For this review, use the dimensioned drawing (mm, ordinates from the lowest corner) and the shaded views. A direction names the side the tool comes from. Coordinates: 2 decimals unless noted, no trailing zeros. Loops run counter-clockwise (first coordinate to the right, second up) from the corner with the lowest first, then second, coordinate; pieces in that order, holes last. Notation, with made-up numbers: M 18,87.25 L 36,87.25 A21 cw 36,92.25 Z; hole C -14,-5.75 d5. An arc over 180 degrees is marked long. Write item = value, one per line. Start each with the question number.
Q1. We need section A-A on z = 30. Give the boundary of the cut face in (x, y), and give its area (3 significant figures).
Q2. Mouldability with a two-part tool opening along Z and no side actions: class the marked faces 5, 6 and 7 as released by +Z, released by -Z, zero draft, split by the parting line, or undercut.
Q3. Wall thickness on probe 1 along Z at (x, y) = (83.5, 7.5); probe 2 along Z at (x, y) = (64.5, 8.25); probe 3 along X at (y, z) = (8.75, 22): over which ranges is each line inside the solid? List them lowest first.
Q4. For the marked faces 1, 2, 3 and 4, list the 3-axis set-ups (+Z, -Z, +X, -X, +Y, -Y) from which the entire face can be reached by the end or side of a thin tool; tool diameter is ignored.
Q5. We need section D-D on x = 9.5. Give the boundary of the cut face in (y, z), and give its area (3 significant figures).
Q6. We need section B-B on y = 4.5. Give the boundary of the cut face in (x, z), and give its area (3 significant figures).
Q7. We need section C-C on x = 42.5. Give the boundary of the cut face in (y, z), and give its area (3 significant figures).
Q8. Clearance check with flat-ended pins moving along their axes: pin 1 Ø13 at (x, z) = (91.5, 21) entering from +Y; pin 2 Ø2.5 at (x, y) = (89.5, 2.5) entering from +Z; pin 3 Ø4 at (x, z) = (89, 18.5) entering from -Y. State where each tip first meets the part, or that it passes through.
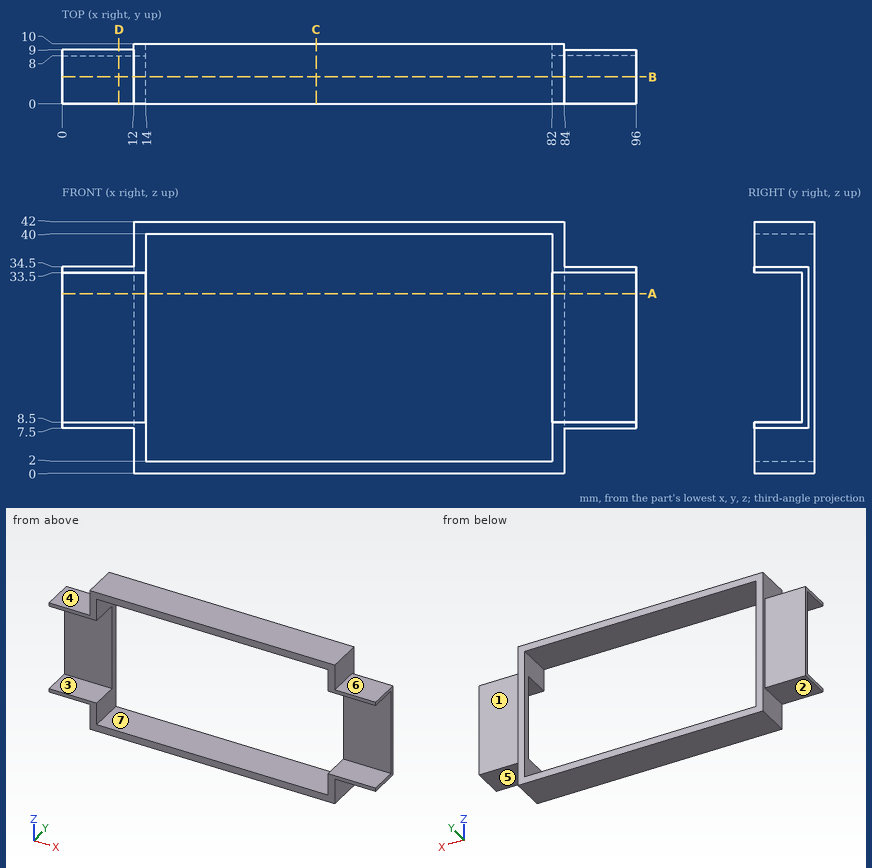
Returned:
q1.outline = M 0,8 L 14,8 L 14,10 L 12,10 L 12,9 L 0,9 Z; M 82,8 L 96,8 L 96,9 L 84,9 L 84,10 L 82,10 Z
q1.area = 32.0 mm^2
q2.face_5 = released by -Z
q2.face_6 = released by +Z
q2.face_7 = undercut
q3.probe_1 = 0 to 8.5, 33.5 to 42
q3.probe_2 = 0 to 2, 40 to 42
q3.probe_3 = 0 to 14, 82 to 96
q4.face_1 = +Z, -Z, +X, +Y
q4.face_2 = -Z, -X, +Y, -Y
q4.face_3 = +X, -X, -Y
q4.face_4 = +Z, -X, +Y, -Y
q5.outline = M 0,7.5 L 9,7.5 L 9,34.5 L 0,34.5 L 0,33.5 L 8,33.5 L 8,8.5 L 0,8.5 Z
q5.area = 43.0 mm^2
q6.outline = M 0,7.5 L 12,7.5 L 12,0 L 84,0 L 84,7.5 L 96,7.5 L 96,8.5 L 82,8.5 L 82,2 L 14,2 L 14,8.5 L 0,8.5 Z; M 0,33.5 L 14,33.5 L 14,40 L 82,40 L 82,33.5 L 96,33.5 L 96,34.5 L 84,34.5 L 84,42 L 12,42 L 12,34.5 L 0,34.5 Z
q6.area = 388 mm^2
q7.outline = M 0,0 L 10,0 L 10,2 L 0,2 Z; M 0,40 L 10,40 L 10,42 L 0,42 Z
q7.area = 40.0 mm^2
q8.pin_1 = 9
q8.pin_2 = 34.5
q8.pin_3 = 8
